```python
from build123d import *

# Parameters (mm, degrees)
PAD_DEPTH    = 3.175
PAD001_DEPTH = 1.905


with BuildPart() as part:
    # Sketch → Pad (new body)
    with BuildSketch(Plane.XY):
        with BuildLine():
            Line((-30.1625, -16.4465), (-30.1625, 16.4465))
            ThreePointArc((-23.9395, 22.6695), (-28.339825, 20.846825), (-30.1625, 16.4465))
            Line((-23.9395, 22.6695), (23.9395, 22.6695))
            ThreePointArc((30.1625, 16.4465), (28.339825, 20.846825), (23.9395, 22.6695))
            Line((30.1625, 16.4465), (30.1625, -16.4465))
            ThreePointArc((23.9395, -22.6695), (28.339825, -20.846825), (30.1625, -16.4465))
            Line((23.9395, -22.6695), (-23.9395, -22.6695))
            ThreePointArc((-30.1625, -16.4465), (-28.339825, -20.846825), (-23.9395, -22.6695))
        make_face()
    extrude(amount=PAD_DEPTH)

    # Sketch001 (on Face10 of Pad) → Pad001 (join)
    with BuildSketch(Plane.XY.offset(3.175)):
        with BuildLine():
            Line((30.1625, -9.4615), (30.1625, 9.4615))
            Line((30.1625, 9.4615), (37.6555, 9.4615))
            Line((37.6555, 9.4615), (37.6555, 1.5875))
            Line((36.068, 1.5875), (37.6555, 1.5875))
            ThreePointArc((36.068, 1.5875), (34.4805, 0), (36.068, -1.5875))
            Line((36.068, -1.5875), (37.6555, -1.5875))
            Line((37.6555, -1.5875), (37.6555, -9.4615))
            Line((37.6555, -9.4615), (30.1625, -9.4615))
        make_face()
        with BuildLine():
            Line((-37.6555, -9.4615), (-37.6555, -1.5875))
            Line((-36.068, -1.5875), (-37.6555, -1.5875))
            ThreePointArc((-36.068, -1.5875), (-34.4805, 0), (-36.068, 1.5875))
            Line((-36.068, 1.5875), (-37.6555, 1.5875))
            Line((-37.6555, 1.5875), (-37.6555, 9.4615))
            Line((-37.6555, 9.4615), (-30.1625, 9.4615))
            Line((-30.1625, 9.4615), (-30.1625, -9.4615))
            Line((-30.1625, -9.4615), (-37.6555, -9.4615))
        make_face()
    extrude(amount=-PAD001_DEPTH)


solid = part.part
```
Design review of the part built by this model. Coordinates are the model's own, in mm. A direction names the side the tool comes from. Coordinates: 2 decimals unless noted, no trailing zeros. Write each loop counter-clockwise with the first axis right and the second up, starting at its lowest first coordinate (ties: lowest second). Pieces come first, ordered by that corner, then holes.
1) Insertion check: pin 1 (1 mm diameter, centred on x = -33, z = 2, fed in from +Y); pin 2 (1.3 mm diameter, centred on x = 36.5, z = 2.5, fed in from -Y); pin 3 (1 mm diameter, centred on y = 12.5, z = 2.5, fed in from +X). Each pin has a flat end and moves straight along its axis. Give the tip position at first contact, or say it passes through.
2) Add section A-A (y = 7.5). Write out the cut boundary in (x, z) (1 decimal), plus the area to 3 significant figures.
3) To check wall thickness, follow L1, parallel to X at y = 5.5, z = 1.1; L2, parallel to Z at x = 33, y = 5.5 (3 decimals); L3, parallel to X at y = -18, z = 0.8. State the ranges of each line that lie inside material, in increasing order.
4) Add section D-D (y = -15). Write out the cut boundary in (x, z) (1 decimal), plus the area to 3 significant figures.
5) Add section B-B (z = 2.4). Write out the cut boundary in (x, y) (1 decimal).
6) Add section C-C (y = 0). Write out the cut boundary in (x, z) (1 decimal).
7) Machinability: for faces 1 (the flat face through (-34, 9.462, 2)), 2 (the flat face through (37, -1.588, 2)), 3 (the flat face through (-37, -1.588, 2)), which of the approach directions +Z, -Z, +X, -X, +Y, -Y give a long, thin tool a straight path to every point of the face, cutting with its end or side? Answer none if there is none.
Check result:
1. pin 1: stops at y = 9.46
1. pin 2: stops at y = -9.46
1. pin 3: stops at x = 30.16
2. outline: (-37.7, 1.3) - (-30.2, 1.3) - (-30.2, 0) - (30.2, 0) - (30.2, 1.3) - (37.7, 1.3) - (37.7, 3.2) - (-37.7, 3.2) - close
2. area: 220 mm2
3. L1: x = -30.16 to 30.16
3. L2: z = 1.27 to 3.175
3. L3: x = -29.97 to 29.97
4. outline: (-30.2, 0) - (30.2, 0) - (30.2, 3.2) - (-30.2, 3.2) - close
4. area: 192 mm2
5. outline: (-37.7, -9.5) - (-30.2, -9.5) - (-30.2, -16.4) arc R6.2 ccw to (-23.9, -22.7) - (23.9, -22.7) arc R6.2 ccw to (30.2, -16.4) - (30.2, -9.5) - (37.7, -9.5) - (37.7, -1.6) - (36.1, -1.6) arc R1.6 cw to (36.1, 1.6) - (37.7, 1.6) - (37.7, 9.5) - (30.2, 9.5) - (30.2, 16.4) arc R6.2 ccw to (23.9, 22.7) - (-23.9, 22.7) arc R6.2 ccw to (-30.2, 16.4) - (-30.2, 9.5) - (-37.7, 9.5) - (-37.7, 1.6) - (-36.1, 1.6) arc R1.6 cw to (-36.1, -1.6) - (-37.7, -1.6) - close
6. outline: (-34.5, 1.3) - (-30.2, 1.3) - (-30.2, 0) - (30.2, 0) - (30.2, 1.3) - (34.5, 1.3) - (34.5, 3.2) - (-34.5, 3.2) - close
7. face 1: +Z, -Z, -X, +Y
7. face 2: +Z, -Z, +X
7. face 3: +Z, -Z, -X
